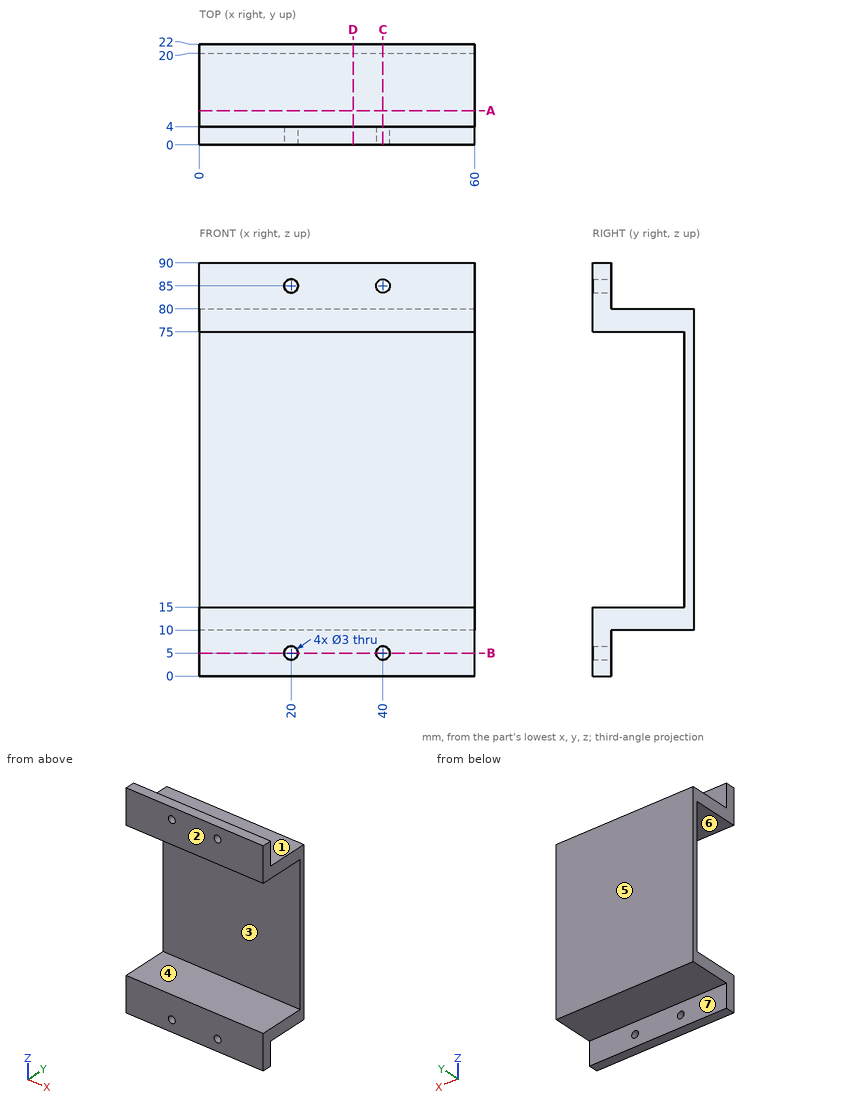
The drawing under review shows one solid part. Ordinate dimensions are in mm from its lowest x, y, z. A direction names the side the tool comes from. Coordinates: 2 decimals unless noted, no trailing zeros. Loops run counter-clockwise (first coordinate to the right, second up) from the corner with the lowest first, then second, coordinate; pieces in that order, holes last. Notation, with made-up numbers: (-18, 39.5) -> (10, 39.5) arc R30 cw to (10, 70.5) -> close; hole circle Ø2 at (-28, 37). An arc over 180 degrees is marked (long way). Answer as a JSON object with one key per item and string values.
Q1. Take a section at B-B on z = 5. Give the boundary of the cut face in (x, y).
Answer block:
{"outline": "(0, 0) -> (18.5, 0) -> (18.5, 4) -> (0, 4) -> close; (21.5, 0) -> (38.5, 0) -> (38.5, 4) -> (21.5, 4) -> close; (41.5, 0) -> (60, 0) -> (60, 4) -> (41.5, 4) -> close"}
Q2. To check wall thickness, follow L1, parallel to X at y = 2.25, z = 85; L2, parallel to Z at x = 20, y = 1.6; L3, parallel to Z at x = 16, y = 16.5. State the ranges of each line that lie inside material, in increasing order.
Answer block:
{"L1": "x = 0 to 18.5, 21.5 to 38.5, 41.5 to 60", "L2": "z = 0 to 3.5, 6.5 to 15, 75 to 83.5, 86.5 to 90", "L3": "z = 10 to 15, 75 to 80"}
Q3. Clearance check with flat-ended pins moving along their axes: pin 1 Ø1 at (x, y) = (16, 12) entering from -Z; pin 2 Ø3 at (x, y) = (39, 12) entering from +Z; pin 3 Ø3 at (x, z) = (26.5, 83) entering from +Y. State where each tip first meets the part, or that it passes through.
Answer block:
{"pin 1": "stops at z = 10", "pin 2": "stops at z = 80", "pin 3": "stops at y = 4"}
Q4. The part is to be moulded in two halves that separate along Z. For the marked faces 1, 2, 3 and 4, say which applies: +Z half, -Z half, draft (parallel to the pull), parting line (faces both ways), or undercut.
Answer block:
{"face 1": "+Z half", "face 2": "draft", "face 3": "undercut", "face 4": "undercut"}
Q5. Take a section at D-D on x = 33.5. Give the boundary of the cut face in (y, z).
Answer block:
{"outline": "(0, 0) -> (4, 0) -> (4, 10) -> (22, 10) -> (22, 80) -> (4, 80) -> (4, 90) -> (0, 90) -> (0, 75) -> (20, 75) -> (20, 15) -> (0, 15) -> close"}
Q6. Take a section at A-A on y = 7.5. Give the boundary of the cut face in (x, z), plus the area to 3 significant figures.
Answer block:
{"outline": "(0, 10) -> (60, 10) -> (60, 15) -> (0, 15) -> close; (0, 75) -> (60, 75) -> (60, 80) -> (0, 80) -> close", "area": "600 mm^2"}
Q7. Tool access review of the marked faces 5, 6 and 7: name each direction out of +Z, -Z, +X, -X, +Y, -Y from which nothing blocks a thin tool from reaching the whole face with its end or side.
Answer block:
{"face 5": "+Z, -Z, +X, -X, +Y", "face 6": "+X, -X, -Y", "face 7": "-Z, +X, -X, +Y"}
Q8. Take a section at C-C on x = 40. Give the boundary of the cut face in (y, z), plus the area to 3 significant figures.
Answer block:
{"outline": "(0, 0) -> (4, 0) -> (4, 3.5) -> (0, 3.5) -> close; (0, 6.5) -> (4, 6.5) -> (4, 10) -> (22, 10) -> (22, 80) -> (4, 80) -> (4, 83.5) -> (0, 83.5) -> (0, 75) -> (20, 75) -> (20, 15) -> (0, 15) -> close; (0, 86.5) -> (4, 86.5) -> (4, 90) -> (0, 90) -> close", "area": "396 mm^2"}
